Could you check a few things on this model? Use its own coordinates, in mm. Face numbers are marked on the shaded views. A direction names the side the tool comes from. Give positions to 0.01 mm unless a question says otherwise; leave off trailing zeros. Loops run counter-clockwise (first coordinate to the right, second up) from the corner with the lowest first, then second, coordinate; pieces in that order, holes last. Notation, with made-up numbers: (88.25, 62.25) -> (145.25, 62.25) arc R12 ccw to (145.25, 80.25) -> close; hole circle Ø1 at (75.5, 60). An arc over 180 degrees is marked (long way). Put each result on its own line as item: value.
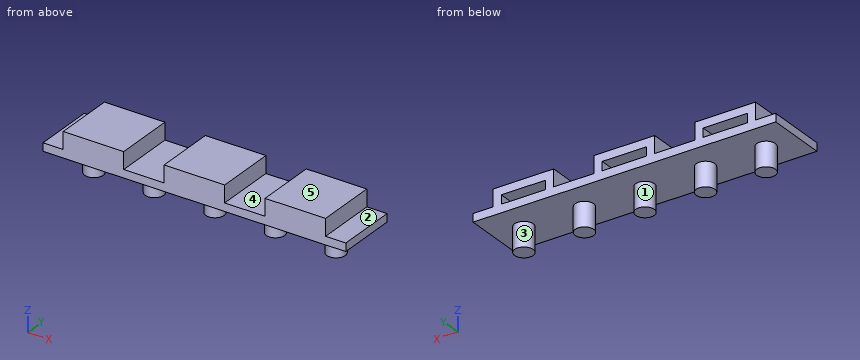
```python
from build123d import *

# Parameters (mm, degrees)
F0_W     = 15
F0_H     = 15
F0_R     = 2.3
F1_DEPTH = 2
F2_DEPTH = 8
F4_DEPTH = 7.5
F5_START = 5.5
F3_W     = 11
F3_H     = 2.2
F5_DEPTH = 2


# Not quite as in the source:
# - a feature names something its author has since deleted; it is built from what else it names


with BuildPart() as f1:
    # F0 (on Top) → F1 (new body)
    with BuildSketch(Plane.XY):
        with Locations((-30, 0)):
            Rectangle(F0_W, F0_H)
        with Locations((-30, 0)):
            Circle(F0_R, mode=Mode.SUBTRACT)
        with Locations((-15, 0)):
            Rectangle(F0_W, F0_H)
        with Locations((-15, 0)):
            Circle(F0_R, mode=Mode.SUBTRACT)
        Rectangle(F0_W, F0_H)
        Circle(F0_R, mode=Mode.SUBTRACT)
        with Locations((15, 0)):
            Rectangle(F0_W, F0_H)
        with Locations((15, 0)):
            Circle(F0_R, mode=Mode.SUBTRACT)
        with Locations((30, 0)):
            Rectangle(F0_W, F0_H)
        with Locations((30, 0)):
            Circle(F0_R, mode=Mode.SUBTRACT)
    extrude(amount=-F1_DEPTH)

    # F0 (on Top) → F2 (join)
    with BuildSketch(Plane.XY):
        with Locations((-15, 0)):
            Circle(F0_R)
        with Locations((-30, 0)):
            Circle(F0_R)
        Circle(F0_R)
        with Locations((15, 0)):
            Circle(F0_R)
        with Locations((30, 0)):
            Circle(F0_R)
    extrude(amount=-F2_DEPTH)

    # F3 (on Front) → F4 (join, symmetric)
    with BuildSketch(Plane.XZ):
        Polygon((-32.5, 4.2), (-32.5, 0), (-30.5, 0), (-30.5, 2.2), (-19.5, 2.2), (-19.5, 0), (-17.5, 0), (-17.5, 4.2), align=None)
        Polygon((5.5, 2.2), (5.5, 0), (7.5, 0), (7.5, 4.2), (-7.5, 4.2), (-7.5, 0), (-5.5, 0), (-5.5, 2.2), align=None)
        Polygon((30.5, 2.2), (30.5, 0), (32.5, 0), (32.5, 4.2), (17.5, 4.2), (17.5, 0), (19.5, 0), (19.5, 2.2), align=None)
    extrude(amount=F4_DEPTH, both=True)

    # F3 (on Front) → F5 (join)
    with BuildSketch(Plane.XZ.offset(F5_START)):
        with Locations((-25, 1.1)):
            Rectangle(F3_W, F3_H)
        with Locations((0, 1.1)):
            Rectangle(F3_W, F3_H)
        with Locations((25, 1.1)):
            Rectangle(F3_W, F3_H)
    extrude(amount=F5_DEPTH)


solid = f1.part
```
1. If we section it at C-C (y = -6.25): List the corners of the cut face in (x, z) for me, then the cut area to 3 significant figures.
Recorded:
outline: (-37.5, -2) -> (37.5, -2) -> (37.5, 0) -> (32.5, 0) -> (32.5, 4.2) -> (17.5, 4.2) -> (17.5, 0) -> (7.5, 0) -> (7.5, 4.2) -> (-7.5, 4.2) -> (-7.5, 0) -> (-17.5, 0) -> (-17.5, 4.2) -> (-32.5, 4.2) -> (-32.5, 0) -> (-37.5, 0) -> close
area: 339 mm^2
2. Thinking about a two-plate mould opening in X: for the marked faces 1 and 2, which applies, pulls with the +X half, pulls with the -X half, needs draft (parallel to the pull), parting line crosses it, or undercut?
Recorded:
face 1: undercut
face 2: needs draft
3. If we section it at D-D (x = -15): List the corners of the cut face in (y, z) for me, then the cut area to 3 significant figures.
Recorded:
outline: (-7.5, -2) -> (-2.3, -2) -> (-2.3, -8) -> (2.3, -8) -> (2.3, -2) -> (7.5, -2) -> (7.5, 0) -> (-7.5, 0) -> close
area: 57.6 mm^2
4. If we section it at A-A (y = 5.5): List the corners of the cut face in (x, z) for me.
Recorded:
outline: (-37.5, -2) -> (37.5, -2) -> (37.5, 0) -> (32.5, 0) -> (32.5, 4.2) -> (17.5, 4.2) -> (17.5, 0) -> (7.5, 0) -> (7.5, 4.2) -> (-7.5, 4.2) -> (-7.5, 0) -> (-17.5, 0) -> (-17.5, 4.2) -> (-32.5, 4.2) -> (-32.5, 0) -> (-37.5, 0) -> close; hole (-30.5, 0) -> (-19.5, 0) -> (-19.5, 2.2) -> (-30.5, 2.2) -> close; hole (-5.5, 0) -> (5.5, 0) -> (5.5, 2.2) -> (-5.5, 2.2) -> close; hole (19.5, 0) -> (30.5, 0) -> (30.5, 2.2) -> (19.5, 2.2) -> close
5. For the marked faces 3, 4 and 5, which set-ups out of +Z, -Z, +X, -X, +Y, -Y let a thin tool reach every point of the face, with its end or its side?
Recorded:
face 3: -Z
face 4: +Z, +Y, -Y
face 5: +Z, +X, -X, +Y, -Y
6. I'm going to push flat-ended pins straight in: pin 1 (6 mm diameter, centred on x = -9, y = 0.5, fed in from -Z); pin 2 (2 mm diameter, centred on x = 0, z = -6.5, fed in from +Y); pin 3 (1.8 mm diameter, centred on y = 0, z = 1, fed in from +X). Where does each tip first touch, or does it pass through?
Recorded:
pin 1: stops at z = -2
pin 2: stops at y = 2.3
pin 3: stops at x = 32.5
7. If we section it at B-B (x = 0): List the corners of the cut face in (y, z) for me, then the cut area to 3 significant figures.
Recorded:
outline: (-7.5, -2) -> (-2.3, -2) -> (-2.3, -8) -> (2.3, -8) -> (2.3, -2) -> (7.5, -2) -> (7.5, 0) -> (-5.5, 0) -> (-5.5, 2.2) -> (7.5, 2.2) -> (7.5, 4.2) -> (-7.5, 4.2) -> close
area: 92.0 mm^2
8. I need wall thicknesses on line 1 (X direction, y = -5.75, z = 2.5); line 2 (Z direction, x = 5, y = -4.5); line 3 (Z direction, x = -29, y = -1.75). Which ranges of each line are inside material? Lowest first, please.
Recorded:
line 1: x = -32.5 to -17.5, -7.5 to 7.5, 17.5 to 32.5
line 2: z = -2 to 0, 2.2 to 4.2
line 3: z = -8 to 0, 2.2 to 4.2
